Source: CAD feature listing. Evaluate the final solid. Frame: model axes, mm. A direction names the side the tool comes from. Give positions to 0.01 mm unless a question says otherwise; leave off trailing zeros. Order: outer loops, then holes, each group sorted by start corner. A loop starts at its lowest first (then second) coordinate and runs counter-clockwise, first axis right, second up. Notation, with made-up numbers: (-3, 72) - (2, 72) arc R9 cw to (2, 79) - close; hole circle Ø11 at (-12, 19.25). An arc over 180 degrees is marked (long way). Answer as CSV lines item,"result".
```python
from build123d import *

# Parameters (mm, degrees)
SKETCH1_R           = 4.15
BOSS_EXTRUDE1_DEPTH = 10
CHAMFER1_SIZE       = 1
CHAMFER1_SIZE2      = 2.747477419


with BuildPart() as part:
    # Sketch1 → Boss-Extrude1 (new body)
    with BuildSketch(Plane(origin=(0, 0, 0), x_dir=(1, 0, 0), z_dir=(0, 1, 0))):
        with BuildLine():
            Line((-39.53507936, 5), (-5, 5))
            Line((-5, 5), (-5, 39.53507936))
            ThreePointArc((-5, 39.53507936), (0, 39.85), (5, 39.53507936))
            Line((5, 39.53507936), (5, 5))
            Line((5, 5), (39.53507936, 5))
            ThreePointArc((39.53507936, 5), (39.85, 0), (39.53507936, -5))
            Line((39.53507936, -5), (5, -5))
            Line((5, -5), (5, -39.53507936))
            ThreePointArc((5, -39.53507936), (0, -39.85), (-5, -39.53507936))
            Line((-5, -39.53507936), (-5, -5))
            Line((-5, -5), (-39.53507936, -5))
            ThreePointArc((-39.53507936, -5), (-39.85, 0), (-39.53507936, 5))
        make_face()
        with Locations(Location((0, 0, 0), (0, 0, 270))):  # turned: the seam where the file's is
            Circle(SKETCH1_R, mode=Mode.SUBTRACT)
    extrude(amount=BOSS_EXTRUDE1_DEPTH)

    # Chamfer1
    chamfer1_edges = [part.edges().sort_by_distance(p)[0] for p in [
        (39.85, 0, 0),
        (0, 0, 39.85),
        (-39.85, 0, 0),
        (0, 0, -39.85),
    ]]
    chamfer1_side = [part.faces().sort_by_distance(p)[0] for p in [
        (-22.26753968, 0, -3.872871791),
    ]]
    chamfer(chamfer1_edges, length=CHAMFER1_SIZE, length2=CHAMFER1_SIZE2, reference=chamfer1_side[0])


solid = part.part
```
(1) Cut plane D-D (z = 17). Return loops of the section in (x, y).
Completed:
outline,"(-5, 0) - (5, 0) - (5, 10) - (-5, 10) - close"
(2) Cut plane A-A (z = 0). Return loops of the section in (x, y).
Completed:
outline,"(-39.85, 2.75) - (-38.85, 0) - (-4.15, 0) - (-4.15, 10) - (-39.85, 10) - close; (4.15, 0) - (38.85, 0) - (39.85, 2.75) - (39.85, 10) - (4.15, 10) - close"
(3) Ray query, line 1 (X direction, y = 3.5, z = 0); line 2 (X direction, y = 6.5, z = -33.5). Return the intervals inside material, ascending. Write a range as from..to.
Completed:
line 1,"-39.85..-4.15, 4.15..39.85"
line 2,"-5..5"
(4) Mould query, pull axis X, two halves, no side actions, for faces 5 (the conical face through (-0.071, 1.393, -39.357)), 6 (the cylindrical face through (-2.53, 4.93, -3.29)), 7 (the flat face through (5, 5, -23)). Classes: released by +X, released by -X, zero draft, split by the parting line, or undercut.
Completed:
face 5,"split by the parting line"
face 6,"undercut"
face 7,"released by +X"
(5) Cut plane B-B (x = 0). Return loops of the section in (y, z), then the cut area to 3 significant figures.
Completed:
outline,"(0, -38.85) - (2.75, -39.85) - (10, -39.85) - (10, -4.15) - (0, -4.15) - close; (0, 4.15) - (10, 4.15) - (10, 39.85) - (2.75, 39.85) - (0, 38.85) - close"
area,"711 mm²"
(6) Cut plane C-C (y = 4.25). Return loops of the section in (x, z), then the cut area to 3 significant figures.
Completed:
outline,"(-39.54, -5) - (-5, -5) - (-5, -39.54) arc R39.85 ccw to (5, -39.54) - (5, -5) - (39.54, -5) arc R39.85 ccw to (39.54, 5) - (5, 5) - (5, 39.54) arc R39.85 ccw to (-5, 39.54) - (-5, 5) - (-39.54, 5) arc R39.85 ccw to start; hole circle Ø8.3 at (0, 0)"
area,"1,440 mm²"
(7) Access query for faces 1 (the flat face through (-23, 5, -5)), 2 (the flat face through (-22, 5, 5)), 3 (the flat face through (22, 5, -5)), 4 (the flat face through (5, 5, 22)). Directions: +Z, -Z, +X, -X, +Y, -Y. A direction counts if a zero-diameter tool reaches every point of the face in a straight line with its end or side. Return the directions, or none.
Completed:
face 1,"-Z, -X, +Y, -Y"
face 2,"+Z, -X, +Y, -Y"
face 3,"-Z, +X, +Y, -Y"
face 4,"+Z, +X, +Y, -Y"
(8) Contact query for flat-ended pins moving along their axis: pin 1 (3 mm diameter, centred on y = 7.5, z = 16.5, fed in from +X); pin 2 (5 mm diameter, centred on x = 12.5, y = 2.5, fed in from +Z); pin 3 (5 mm diameter, centred on x = -25.5, y = 6.5, fed in from -Z). Output: stop coordinate, or through.
Completed:
pin 1,"x = 5"
pin 2,"z = 5"
pin 3,"z = -5"
